Read the model definition and answer for the solid it produces. Units are mm, in the model's axes. Face numbers are marked on the shaded views. A direction names the side the tool comes from. Coordinates: 2 decimals unless noted, no trailing zeros. Loops run counter-clockwise (first coordinate to the right, second up) from the corner with the lowest first, then second, coordinate; pieces in that order, holes last.
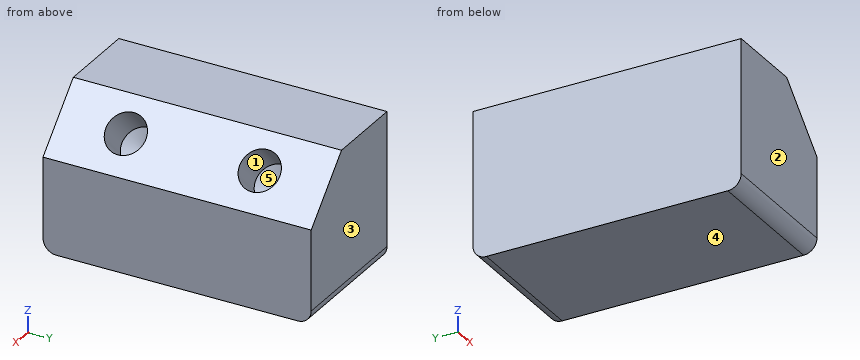
from build123d import *

# Parameters (mm, degrees)
F0_W     = 50
F0_H     = 100
F1_DEPTH = 55
F2_SIZE  = 20
F4_D     = 15
F4_DEPTH = 15
F4_TIP   = 4.5064546427
F6_D     = 15
F6_DEPTH = 15
F6_TIP   = 4.5064546427
F8_R     = 5
F9_R     = 5


with BuildPart() as f1:
    # F0 (on Top) → F1 (new body)
    with BuildSketch(Plane.XY):
        with Locations((25, 50)):
            Rectangle(F0_W, F0_H)
    extrude(amount=F1_DEPTH)

    # F2
    f2_edges = [f1.edges().sort_by_distance(p)[0] for p in [
        (50, 50, 55),
    ]]
    chamfer(f2_edges, length=F2_SIZE)

    # F4
    with Locations(Plane(origin=(42.5, 0, 42.5), x_dir=(0.7071067812, 0, -0.7071067812), z_dir=(0.7071067812, 0, 0.7071067812))):
        with Locations((-4.1437726468, 25)):
            Hole(F4_D / 2, depth=F4_DEPTH)
            with Locations((0, 0, -(F4_DEPTH + F4_TIP / 2))):  # 118° drill point
                Cone(0, F4_D / 2, F4_TIP, mode=Mode.SUBTRACT)

    # F6
    with Locations(Plane(origin=(42.5, 0, 42.5), x_dir=(0.7071067812, 0, -0.7071067812), z_dir=(0.7071067812, 0, 0.7071067812))):
        with Locations((-3.94243747, 75)):
            Hole(F6_D / 2, depth=F6_DEPTH)
            with Locations((0, 0, -(F6_DEPTH + F6_TIP / 2))):  # 118° drill point
                Cone(0, F6_D / 2, F6_TIP, mode=Mode.SUBTRACT)

    # F8
    f8_edges = [f1.edges().sort_by_distance(p)[0] for p in [
        (25, 100, 0),
    ]]
    fillet(f8_edges, radius=F8_R)

    # F9
    f9_edges = [f1.edges().sort_by_distance(p)[0] for p in [
        (25, 0, 0),
    ]]
    fillet(f9_edges, radius=F9_R)


solid = f1.part
Q1. Straight lines are drawn through the part: probe 1 along Z at (x, y) = (39, 25.5); probe 2 along Y at (x, z) = (29.5, 42); probe 3 along Z at (x, y) = (29, 26). For each, find the intervals that lie inside material, in ascending order.
Findings below:
probe 1: z = 0 to 34.28
probe 2: y = 0 to 19.15, 30.85 to 69.32, 80.68 to 100
probe 3: z = 0 to 30.93, 45.37 to 55
Q2. A cutting plane is placed at A-A (y = 41). Give the vertices of the cut face in (x, z).
Findings below:
outline: (0, 0) - (50, 0) - (50, 35) - (30, 55) - (0, 55) - close
Q3. Determine the mould class of the marked faces 1, 2 and 3 for opening direction Y: +Y half, -Y half, draft (parallel to the pull), parting line (faces both ways), or undercut.
Findings below:
face 1: undercut
face 2: -Y half
face 3: +Y half
Q4. Which of the six approach directions +Z, -Z, +X, -X, +Y, -Y give full straight-line access (tool end or side, diameter ignored) to the marked faces 4 and 5?
Findings below:
face 4: -Z, +X, -X, +Y, -Y
face 5: none
Q5. Flat-ended cylindrical pins translate along their axes: pin 1 Ø4 at (y, z) = (66, 44.5) entering from -X; pin 2 Ø3 at (y, z) = (46.5, 38) entering from +X. Find the tip coordinate at first contact, or state that the pin passes through.
Findings below:
pin 1: stops at x = 0
pin 2: stops at x = 48.5
